Autodesk Inventor part; units mm, degrees
ref_plane "YZ Plane" through (0, 0, 0) normal (1, 0, 0) x (0, 1, 0)
ref_plane "XZ Plane" through (0, 0, 0) normal (0, 1, 0) x (-1, 0, 0)
ref_plane "XY Plane" through (0, 0, 0) normal (0, 0, 1) x (1, 0, 0)
sketch "Sketch12" plane through (0, 0, 0) normal (0, 0, 1) x (1, 0, 0)
  line L0 (0, 0) -> (35, 0)
  line L1 (35, 0) -> (35, 47)
  line L2 (35, 47) -> (0, 47)
  line L3 (0, 47) -> (0, 0)
  line L4 (0, 47) -> (2, 47) construction
  line L5 (2, 47) -> (2, 35.5) construction
  line L6 (35, 47) -> (33, 47) construction
  line L7 (33, 47) -> (33, 35.5) construction
  circle A0 centre (33, 35.5) radius 1.25
  circle A1 centre (2, 35.5) radius 1.25
  line L8 (0, 0) -> (6.5, 0) construction
  line L9 (35, 0) -> (28.5, 0) construction
  line L10 (6.5, 0) -> (6.5, 3.2) construction
  line L11 (28.5, 0) -> (28.5, 3.2) construction
  circle A2 centre (28.5, 3.2) radius 1.25
  dimension "d49" = 35
  dimension "d50" = 47
  dimension "d97" = 2
  dimension "d98" = 11.5
  dimension "d99" = 2
  dimension "d100" = 2.5
  dimension "d101" = 2.5
  dimension "d102" = 11.5
  dimension "d104" = 6.5
  dimension "d106" = 3.2
  dimension "d108" = 2.5
extrude "Extrusión8" add sketch "Sketch12" along normal blind 1
sketch "Sketch25" plane through (0, 47, 0) normal (0, 1, 0) x (1, 0, 0)
  point P0 (0, 0)
sketch "Sketch27" plane through (0, 0, 0) normal (0, -1, 0) x (1, 0, 0)
  line L0 (0, 0) -> (14.7732, 0)
  line L1 (14.7732, 0) -> (14.7732, -14)
  line L2 (14.7732, -14) -> (0, -14)
  line L3 (0, -14) -> (0, 0)
  dimension "d125" = 14
extrude "Extrusion11" add sketch "Sketch27" against normal blind 1
fillet "Empalme1" radius 2 1 edges at (7.3866, 1, 0)
sketch "Boceto29" plane through (0, 47, 0) normal (0, 1, 0) x (1, 0, 0)
  line L0 (14.7732, 0) -> (14.7732, 2)
  line L1 (0, 0) -> (14.7732, 0)
  line L2 (14.7732, 0) -> (0, 0)
  line L3 (0, 14) -> (0, 2)
  line L4 (0, 0) -> (0, 14)
  line L5 (14.7732, 14) -> (0, 14)
  line L6 (0, 14) -> (14.7732, 14)
  line L7 (14.7732, 14) -> (14.7732, 0)
  point P0 (0, 2)
extrude "Extrusión12" add sketch "Boceto29" against normal blind 1
fillet "Empalme2" radius 2 1 edges at (7.3866, 46, 0)
sketch "Boceto30" plane through (0, 47, 1) normal (0, 1, 0) x (1, 0, 0)
  line L0 (0, 15) -> (0, 0)
  line L1 (0, 7.5) -> (14.7732, 7.5)
  line L2 (14.7732, 15) -> (14.7732, 3)
  line L3 (7.3866, 7.5) -> (7.3866, 0)
  line L4 (35, 0) -> (0, 0)
  circle A0 centre (7.3866, 7.5) radius 1.5
  point P0 (0, 1)
  dimension "d126" = 3
extrude "Extrusión13" cut sketch "Boceto30" along normal through all both and the other way through all contours A0 L1 | L1 L3 A0 | L1 A0 L3
equation "\"BendRadius\" = Thickness"
equation "\"BendReliefWidth\" = Thickness"
equation "\"BendReliefDepth\" = 0.5 * Thickness"
equation "\"CornerReliefSize\" = 4 * Thickness"
equation "\"MinimumRemnant\" = 2 * Thickness"
equation "\"TransitionRadius\" = BendRadius"
equation "\"JacobiRadiusSize\" = BendRadius"
equation "\"GapSize\" = Thickness"
properties part number "Suportmotor"
CAD build for the part. Positions are in the model's coordinates, mm. A direction names the side the tool comes from. Give positions to 0.01 mm unless a question says otherwise; leave off trailing zeros. Write each loop counter-clockwise with the first axis right and the second up, starting at its lowest first coordinate (ties: lowest second). Pieces come first, ordered by that corner, then holes. Notation, with made-up numbers: M -34.5,73 L 23.5,73 A13 cw 23.5,79 Z; hole C -27.5,65 d5. An arc over 180 degrees is marked long. Return JSON: item names as keys, results as strings. Group by question number.
(1) Flat gauge pins, fed straight in: pin 1 Ø3.5 at (y, z) = (1.5, -8) entering from +X; pin 2 Ø17.5 at (x, y) = (22.5, 16.5) entering from -Z; pin 3 Ø12 at (x, y) = (11, 8.5) entering from -Z. Where does each tip first touch, or does it go through?
(2) Band-saw the part on C-C (z = -6.5). Give the cut face in (x, y), and give its area (3 significant figures).
(3) Band-saw the part on D-D (x = 28.5). Give the cut face in (y, z).
(4) Mould opens along Z. For faces 1 (the face through (17, 24, 0)), 2 (the face through (6.196, 46.507, -5.587)), 3 (the face through (0, 23.6, 0.2)) say: pulls with the +Z half, pulls with the -Z half, needs draft (parallel to the pull), parting line crosses it, or undercut.
(5) Band-saw the part on A-A (z = -10.25). Give the cut face in (x, y), and give its area (3 significant figures).
(6) Band-saw the part on B-B (x = 2). Give the cut face in (y, z), and give its area (3 significant figures).
(7) Drill centre lines: L1, parallel to X at y = 0.45, z = -6.5; L2, parallel to Y at x = 14, z = -10.5; L3, parallel to Y at x = 2, z = 0.8. Where is each one in solid material? Low to high. Write a range as [from, to].
(8) 3-axis set-ups, long thin cutter, end or side, ignore diameter. For faces 4 (the face through (14.773, 46.4, -6.5)), 5 (the face through (7, 1, -9)), 6 (the face through (17, 24, 1)): which of +Z, -Z, +X, -X, +Y, -Y reach the whole face in a straight line?
Entries:
{
 "1": {"pin 1": "stops at x = 14.77", "pin 2": "stops at z = 0", "pin 3": "stops at z = -0.06"},
 "2": {"outline": "M 0,0 L 5.89,0 L 5.89,1 L 0,1 Z; M 0,46 L 5.89,46 L 5.89,47 L 0,47 Z; M 8.89,0 L 14.77,0 L 14.77,1 L 8.89,1 Z; M 8.89,46 L 14.77,46 L 14.77,47 L 8.89,47 Z", "area": "23.5 mm^2"},
 "3": {"outline": "M 0,0 L 1.95,0 L 1.95,1 L 0,1 Z; M 4.45,0 L 47,0 L 47,1 L 4.45,1 Z"},
 "4": {"face 1": "pulls with the -Z half", "face 2": "undercut", "face 3": "needs draft"},
 "5": {"outline": "M 0,0 L 14.77,0 L 14.77,1 L 0,1 Z; M 0,46 L 14.77,46 L 14.77,47 L 0,47 Z", "area": "29.5 mm^2"},
 "6": {"outline": "M 0,-14 L 1,-14 L 1,-2 A2 cw 3,0 L 34.25,0 L 34.25,1 L 0,1 Z; M 36.75,0 L 44,0 A2 cw 46,-2 L 46,-14 L 47,-14 L 47,1 L 36.75,1 Z", "area": "74.2 mm^2"},
 "7": {"L1": "x = [0, 5.89], [8.89, 14.77]", "L2": "y = [0, 1], [46, 47]", "L3": "y = [0, 34.25], [36.75, 47]"},
 "8": {"face 4": "-Z, +X, +Y, -Y", "face 5": "-Z, +X, -X", "face 6": "+Z, +X, -X, +Y, -Y"}
}
